Source: CAD feature listing. Evaluate the final solid. Frame: model axes, mm. A direction names the side the tool comes from. Round coordinates to 2 decimals unless told otherwise and drop trailing zeros. Order: outer loops, then holes, each group sorted by start corner. A loop starts at its lowest first (then second) coordinate and runs counter-clockwise, first axis right, second up. Notation, with made-up numbers: (-12.75, 17) - (19.25, 17) arc R16 ccw to (19.25, 41) - close; hole circle Ø8 at (55.5, 73). An arc over 180 degrees is marked (long way). Return JSON: item names as keys, results as strings. Group by question number.
1) Access query for faces 1 (the flat face through (-1.14, 0.63, 1.37)), 2 (the flat face through (-1, -1, 2.2)). Directions: +Z, -Z, +X, -X, +Y, -Y. A direction counts if a zero-diameter tool reaches every point of the face in a straight line with its end or side. Return the directions, or none.
2) Section A-A, the plane z = -29. Return loops of the section in (x, y), plus the area to 3 significant figures.
3) Mould query, pull axis X, two halves, no side actions, for faces 3 (the cylindrical face through (2, 0, -16)), 4 (the flat face through (0, 0, -32.8)), 5 (the flat face through (0.64, -1.16, 1.56)). Classes: pulls with the +X half, pulls with the -X half, needs draft (parallel to the pull), parting line crosses it, or undercut.
4) Ray query, line 1 (X direction, y = -0.75, z = -18.5); line 2 (Z direction, x = -2, y = 2.25); line 3 (X direction, y = 1.5, z = -26.5). Return the intervals inside material, ascending. Write a range as from..to.
5) Contact query for flat-ended pins moving along their axis: P1, Ø2, axis at y = 1.5, z = -8, coming from the -X side; P2, Ø1, axis at x = -2, z = -4.5, coming from the -Y side; P3, Ø3, axis at y = 1, z = -10, coming from the +X side. Output: stop coordinate, or through.
```python
from build123d import *

# Parameters (mm, degrees)
CUT_EXTRUDE1_REACH = 37.4
CIRPATTERN1_COUNT  = 4
DRAFT2_ANGLE       = 5


with BuildPart() as part:
    # Sketch3 → Revolve1 (revolve)
    with BuildSketch(Plane(origin=(0, 0, 0), x_dir=(0, 0, -1), z_dir=(1, 0, 0)), mode=Mode.PRIVATE) as revolve1_sk:
        Polygon((-2.2, 0), (-2.2, 3.75), (-0.45, 2), (-0.45, 0), align=None)
    revolve(revolve1_sk.sketch.rotate(Axis((0, 0, 2.2), (0, 0, -1)), 180), axis=Axis((0, 0, 2.2), (0, 0, -1)))

    # Sketch5 → Revolve2 (revolve)
    with BuildSketch(Plane(origin=(0, 0, 0), x_dir=(0, 0, -1), z_dir=(1, 0, 0))):
        Polygon((32.8, 0), (-0.45, 0), (-0.45, 2), (32.247, 2), (32.8, 1.447), align=None)
    revolve(axis=Axis((0, 0, -32.8), (0, 0, 1)))

    # Cut-Extrude1: up to this cone (the profile starts inside it)
    cut_extrude1_end = Plane(origin=(0, 0, 2.2), z_dir=(0, 0, 1)).offset(-2.704989458) * Cone(1e-06, 43.309980917, 43.309979917, align=(Align.CENTER, Align.CENTER, Align.MIN), mode=Mode.PRIVATE)
    # Sketch4 → Cut-Extrude1 (cut, up to the surface)
    with BuildSketch(Plane.XY.offset(2.2), mode=Mode.PRIVATE) as cut_extrude1_sk1:
        with BuildLine():
            Line((0, 0), (2.6416, 0))
            ThreePointArc((2.6416, 0), (2.627961466, 0.268084114), (2.587186696, 0.5334))
            Line((2.587186696, 0.5334), (1.560293348, 0.5334))
            Line((1.560293348, 0.5334), (0.834170098, 0.834170098))
            Line((0.834170098, 0.834170098), (0.5334, 1.560293348))
            Line((0.5334, 1.560293348), (0.5334, 2.587186696))
            ThreePointArc((0.5334, 2.587186696), (0.268084114, 2.627961466), (0, 2.6416))
            Line((0, 2.6416), (0, 0))
        make_face()
    cut_extrude1_tool1 = extrude(cut_extrude1_sk1.sketch, amount=-CUT_EXTRUDE1_REACH, mode=Mode.PRIVATE) & cut_extrude1_end
    cut_extrude1 = cut_extrude1_tool1.solids().sort_by_distance((0.037358, 1.3208, 2.2))[0]
    add(cut_extrude1, mode=Mode.SUBTRACT)

    # CirPattern1: Cut-Extrude1 ×4 about axis
    cirpattern1_axis = Axis((0, 0, 0), (0, 0, 1))
    for i in range(1, CIRPATTERN1_COUNT):
        add(cut_extrude1.rotate(cirpattern1_axis, i * 360 / CIRPATTERN1_COUNT), mode=Mode.SUBTRACT)

    # Draft2
    draft2_faces = [part.faces().sort_by_distance(p)[0] for p in [
        (-1.92259155, 0.5334, 1.845671202),
        (-1.175407967, 0.692824745, 1.535600175),
        (-0.692824745, 1.175407967, 1.535600175),
        (-0.5334, 1.92259155, 1.845671202),
        (0.5334, 1.92259155, 1.845671202),
        (0.692824745, 1.175407967, 1.535600175),
        (1.175407967, 0.692824745, 1.535600175),
        (1.92259155, 0.5334, 1.845671202),
        (1.92259155, -0.5334, 1.845671202),
        (1.175407967, -0.692824745, 1.535600175),
        (0.692824745, -1.175407967, 1.535600175),
        (0.5334, -1.92259155, 1.845671202),
        (-0.5334, -1.92259155, 1.845671202),
        (-0.692824745, -1.175407967, 1.535600175),
        (-1.175407967, -0.692824745, 1.535600175),
        (-1.92259155, -0.5334, 1.845671202),
    ]]
    draft(draft2_faces, Plane(origin=(0, 0, 2.2), x_dir=(0, 1, 0), z_dir=(0, 0, 1)), DRAFT2_ANGLE)


solid = part.part
```
Geometry check:
{
 "1": {"face 1": "+Z", "face 2": "+Z, +X, -X, +Y, -Y"},
 "2": {"outline": "circle Ø4 at (0, 0)", "area": "12.6 mm2"},
 "3": {"face 3": "parting line crosses it", "face 4": "needs draft", "face 5": "undercut"},
 "4": {"line 1": "-1.85..1.85", "line 2": "1.46..2.2", "line 3": "-1.32..1.32"},
 "5": {"P1": "x = -1.94", "P2": "y = -1.32", "P3": "x = 2"}
}
